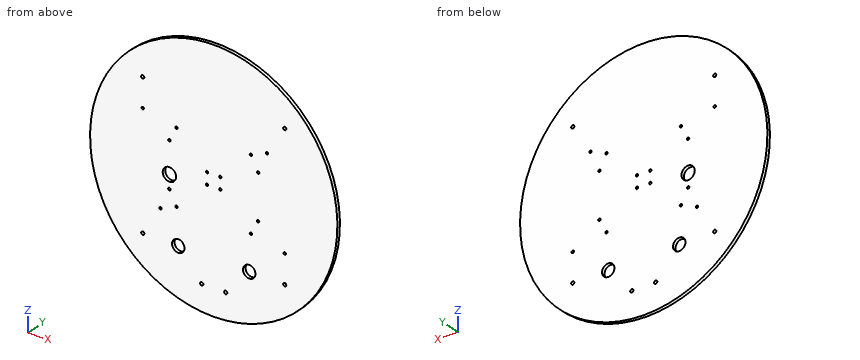
```python
from build123d import *

# Parameters (mm, degrees)
SKETCH1_R            = 177
SKETCH1_R_2          = 2.2479
BOSS_EXTRUDE1_DEPTH  = 4.7625
SKETCH2_R            = 1.7
JETSONHOLES_DEPTH    = 251.361102023
SKETCH3_R            = 9.525
UART_WIRE_HOLE_DEPTH = 4.7625
SKETCH4_R            = 2.286
CAMERA_HOLE_DEPTH    = 4.7625
SKETCH5_R            = 1.7
STANDOFFHOLES_DEPTH  = 251.361102023
SKETCH6_R            = 1.7
SKETCH6_R_2          = 8.89
NIMH_HOLES_DEPTH     = 251.361102023
SKETCH7_R            = 1.7
IMU_HOLES_DEPTH      = 251.361102023


with BuildPart() as part:
    # Sketch1 → Boss-Extrude1 (new body)
    with BuildSketch(Plane(origin=(0, 0, 0), x_dir=(1, 0, 0), z_dir=(0, 1, 0))):
        with Locations(Location((0, 0, 0), (0, 0, 90))):
            Circle(SKETCH1_R)
        with Locations(Location((-101.6, -101.6, 0), (0, 0, 90))):
            Circle(SKETCH1_R_2, mode=Mode.SUBTRACT)
        with Locations(Location((-101.6, 101.6, 0), (0, 0, 90))):
            Circle(SKETCH1_R_2, mode=Mode.SUBTRACT)
        with Locations(Location((101.6, 101.6, 0), (0, 0, 90))):
            Circle(SKETCH1_R_2, mode=Mode.SUBTRACT)
        with Locations(Location((101.6, -101.6, 0), (0, 0, 90))):
            Circle(SKETCH1_R_2, mode=Mode.SUBTRACT)
    extrude(amount=BOSS_EXTRUDE1_DEPTH)

    # Sketch2 → JetsonHoles (cut, through all)
    with BuildSketch(Plane(origin=(0, 4.7625, 0), x_dir=(1, 0, 0), z_dir=(0, 1, 0))):
        with Locations(Location((-53.213, 51.435, 0), (0, 0, 270))):
            Circle(SKETCH2_R)
        with Locations(Location((53.213, 51.435, 0), (0, 0, 270))):
            Circle(SKETCH2_R)
        with Locations(Location((-53.213, -51.435, 0), (0, 0, 270))):
            Circle(SKETCH2_R)
        with Locations(Location((53.213, -51.435, 0), (0, 0, 270))):
            Circle(SKETCH2_R)
    extrude(amount=-JETSONHOLES_DEPTH, mode=Mode.SUBTRACT)

    # Sketch3 → UART-Wire-Hole (cut)
    with BuildSketch(Plane(origin=(0, 4.7625, 0), x_dir=(1, 0, 0), z_dir=(0, 1, 0))):
        with Locations(Location((-63.5, 12.7, 0), (0, 0, 270))):
            Circle(SKETCH3_R)
    extrude(amount=-UART_WIRE_HOLE_DEPTH, mode=Mode.SUBTRACT)

    # Sketch4 → Camera-Hole (cut)
    with BuildSketch(Plane(origin=(0, 4.7625, 0), x_dir=(1, 0, 0), z_dir=(0, 1, 0))):
        with Locations(Location((-17.145, 139.7, 0), (0, 0, 270))):
            Circle(SKETCH4_R)
        with Locations(Location((17.145, 139.7, 0), (0, 0, 270))):
            Circle(SKETCH4_R)
    extrude(amount=-CAMERA_HOLE_DEPTH, mode=Mode.SUBTRACT)

    # Sketch5 → StandoffHoles (cut, through all)
    with BuildSketch(Plane(origin=(0, 4.7625, 0), x_dir=(1, 0, 0), z_dir=(0, 1, 0))):
        with Locations(Location((-63.5, -31.75, 0), (0, 0, 270))):
            Circle(SKETCH5_R)
        with Locations(Location((63.5, -31.75, 0), (0, 0, 270))):
            Circle(SKETCH5_R)
        with Locations(Location((63.5, 31.75, 0), (0, 0, 270))):
            Circle(SKETCH5_R)
        with Locations(Location((-63.5, 31.75, 0), (0, 0, 270))):
            Circle(SKETCH5_R)
    extrude(amount=-STANDOFFHOLES_DEPTH, mode=Mode.SUBTRACT)

    # Sketch6 → NiMH_Holes (cut, through all)
    with BuildSketch(Plane(origin=(0, 4.7625, 0), x_dir=(1, 0, 0), z_dir=(0, 1, 0))):
        with Locations(Location((101.6, 60.96, 0), (0, 0, 270))):
            Circle(SKETCH6_R)
        with Locations(Location((76.2, -60.96, 0), (0, 0, 270))):
            Circle(SKETCH6_R)
        with Locations(Location((-101.6, -60.96, 0), (0, 0, 270))):
            Circle(SKETCH6_R)
        with Locations(Location((-76.2, 60.96, 0), (0, 0, 270))):
            Circle(SKETCH6_R)
        with Locations(Location((-50.8, 101.6, 0), (0, 0, 270))):
            Circle(SKETCH6_R_2)
        with Locations(Location((50.8, 101.6, 0), (0, 0, 270))):
            Circle(SKETCH6_R_2)
    extrude(amount=-NIMH_HOLES_DEPTH, mode=Mode.SUBTRACT)

    # Sketch7 → IMU_Holes (cut, through all)
    with BuildSketch(Plane(origin=(0, 4.7625, 0), x_dir=(1, 0, 0), z_dir=(0, 1, 0))):
        with Locations(Location((-9.55000005, 8.162499942, 0), (0, 0, 270))):
            Circle(SKETCH7_R)
        with Locations(Location((9.54999995, 8.162499942, 0), (0, 0, 270))):
            Circle(SKETCH7_R)
        with Locations(Location((-9.55000005, -8.162500058, 0), (0, 0, 270))):
            Circle(SKETCH7_R)
        with Locations(Location((9.54999995, -8.162500058, 0), (0, 0, 270))):
            Circle(SKETCH7_R)
    extrude(amount=-IMU_HOLES_DEPTH, mode=Mode.SUBTRACT)


solid = part.part
```
Geometry: final body of the model. Coordinates: model frame, mm. Round coordinates to 2 decimals unless told otherwise and drop trailing zeros. Write each loop counter-clockwise with the first axis right and the second up, starting at its lowest first coordinate (ties: lowest second). Pieces come first, ordered by that corner, then holes. Notation, with made-up numbers: (-34.5, 49) -> (-12.5, 49) arc R26 cw to (-12.5, 64) -> close; hole circle Ø5 at (-35, 75.25). An arc over 180 degrees is marked (long way). Use CSV: the item, a comma, the result in double quotes. Start each with the question number.
Q1. Line query: L1, parallel to X at y = 1.5, z = -101.6; L2, parallel to X at y = 0.75, z = -51; L3, parallel to X at y = 0.85, z = -1.5. Output: solid intervals per line, ascending.
Q2. Section B-B (x = -126). Return loops of the section in (y, z), plus the area to 3 significant figures.
Q3. First-contact query: pin 1 Ø2 at (x, y) = (93, 1) entering from +Z. Flat tip, straight axial feed; report the tip coordinate or a pass-through.
Q4. Section A-A (y = 2.65). Give the number of separate pieces and of enclosed holes in the cut face, plus the area to 3 significant figures.
Q5. Section C-C (z = 130.5). Return loops of the section in (x, y), plus the area to 3 significant figures.
Result sheet:
1,L1,"-144.94 to -103.85, -99.35 to -59.69, -41.91 to 41.91, 59.69 to 99.35, 103.85 to 144.94"
1,L2,"-169.49 to -54.86, -51.57 to 51.57, 54.86 to 169.49"
1,L3,"-176.99 to 176.99"
2,outline,"(0, -124.31) -> (4.76, -124.31) -> (4.76, 124.31) -> (0, 124.31) -> close"
2,area,"1,180 mm²"
3,pin 1,"z = 151.21"
4,separate pieces,"1"
4,enclosed holes,"25"
4,area,"97,400 mm²"
5,outline,"(-119.58, 0) -> (119.58, 0) -> (119.58, 4.76) -> (-119.58, 4.76) -> close"
5,area,"1,140 mm²"
